```python
from build123d import *

# Parameters (mm, degrees)
SKETCH1_R           = 2
BOSS_EXTRUDE1_DEPTH = 40
FILLET1_R           = 4


with BuildPart() as part:
    # Sketch1 → Boss-Extrude1 (new body)
    with BuildSketch(Plane.XY):
        with BuildLine():
            Line((-123.999650399, -12.7366), (-133.999632379, -12.755584536))
            ThreePointArc((-133.999632379, -12.755584536), (-126.357727013, -67.682340192), (-104.205340418, -118.521488224))
            Line((-104.205340418, -118.521488224), (-95.406545634, -113.742234823))
            ThreePointArc((-95.406545634, -113.742234823), (-116.664774404, -65.210158377), (-123.999650399, -12.7366))
        make_face()
        with Locations((-128.565543545, -25.510785173)):
            Circle(SKETCH1_R, mode=Mode.SUBTRACT)
        with Locations((-124.80403691, -53.01786585)):
            Circle(SKETCH1_R, mode=Mode.SUBTRACT)
        with Locations((-117.250891281, -79.733748965)):
            Circle(SKETCH1_R, mode=Mode.SUBTRACT)
        with Locations((-106.053120049, -105.138440244)):
            Circle(SKETCH1_R, mode=Mode.SUBTRACT)
    extrude(amount=BOSS_EXTRUDE1_DEPTH)

    # Fillet1
    fillet1_edges = [part.edges().sort_by_distance(p)[0] for p in [
        (-95.406545634, -113.742234823, 20),
    ]]
    fillet(fillet1_edges, radius=FILLET1_R)


solid = part.part
```
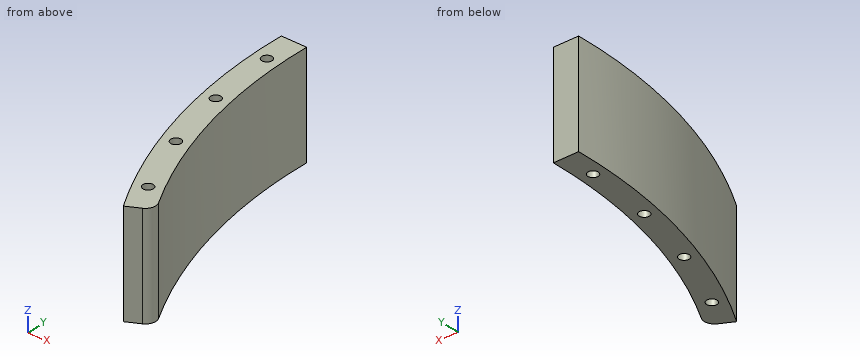
Part model, mm, in its own coordinate system. Give positions to 0.01 mm unless a question says otherwise; leave off trailing zeros. Loops run counter-clockwise (first coordinate to the right, second up) from the corner with the lowest first, then second, coordinate; pieces in that order, holes last. Notation, with made-up numbers: M 71.25,56 L 104.25,56 A22 ccw 104.25,71 Z; hole C 35.5,63 d4. An arc over 180 degrees is marked long. Return JSON: item names as keys, results as strings.
1) Saw through at D-D, the plane x = -117. List the corners of the cut face in (y, z).
Calculated:
{"outline": "M -93.9,0 L -81.72,0 L -81.72,40 L -93.9,40 Z; M -77.75,0 L -64.01,0 L -64.01,40 L -77.75,40 Z"}
2) Drill centre lines: line 1 (Y direction, x = -105, z = 17.5); line 2 (Y direction, x = -107, z = 36); line 3 (Y direction, x = -101, z = 7). Where is each one in solid material? Low to high.
Calculated:
{"line 1": "y = -117.21 to -106.84, -103.44 to -96.1", "line 2": "y = -113.79 to -106.9, -103.38 to -91.78", "line 3": "y = -116.78 to -103.99"}
3) Saw through at B-B, the plane z = 5.5. List the corners of the cut face in (x, y).
Calculated:
{"outline": "M -134,-12.76 A204 ccw -104.21,-118.52 L -99.07,-115.73 A4 ccw -97.53,-110.2 A194 cw -124,-12.74 Z; hole C -128.57,-25.51 d4; hole C -124.8,-53.02 d4; hole C -117.25,-79.73 d4; hole C -106.05,-105.14 d4"}
4) Saw through at C-C, the plane y = -69. List the corners of the cut face in (x, z), then the cut area to 3 significant figures.
Calculated:
{"outline": "M -125.98,0 L -115.55,0 L -115.55,40 L -125.98,40 Z", "area": "417 mm2"}
5) Saw through at A-A, the plane x = -125.5. List the corners of the cut face in (y, z), then the cut area to 3 significant figures.
Calculated:
{"outline": "M -70.64,0 L -54.89,0 L -54.89,40 L -70.64,40 Z; M -51.14,0 L -12.74,0 L -12.74,40 L -51.14,40 Z", "area": "2,170 mm2"}
6) Flat gauge pins, fed straight in: pin 1 Ø4 at (x, z) = (-111, 27.5) entering from -Y; pin 2 Ø4 at (y, z) = (-62.5, 20) entering from -X; pin 3 Ø12 at (y, z) = (-45.5, 12.5) entering from +X. Where does each tip first touch, or does it go through?
Calculated:
{"pin 1": "stops at y = -110.22", "pin 2": "stops at x = -128.24", "pin 3": "stops at x = -120.01"}
